The listing builds one solid part. Answer for the finished solid, in the listing's coordinates (mm). Round coordinates to 2 decimals unless told otherwise and drop trailing zeros. Loops run counter-clockwise (first coordinate to the right, second up) from the corner with the lowest first, then second, coordinate; pieces in that order, holes last. Notation, with made-up numbers: M 75,-14.5 L 93,-14.5 A12 ccw 93,-4.5 Z; hole C 47,88.25 d1. An arc over 180 degrees is marked long. Answer as a JSON object with one key per item and string values.
```python
from build123d import *

# Parameters (mm, degrees)
SKETCH1_W               = 10
SKETCH1_H               = 6
BOSS_EXTRUDE1_DEPTH     = 250
SKETCH3_R               = 3
CUT_EXTRUDE2_DEPTH      = 249
CUT_EXTRUDE2_DEPTH_BACK = 249
SKETCH2_W               = 8
SKETCH2_H               = 4
CUT_EXTRUDE4_DEPTH      = 251
CUT_EXTRUDE4_DEPTH_BACK = 1
SKETCH7_R               = 6
BOSS_EXTRUDE2_DEPTH     = 10
SKETCH9_R               = 5
CUT_EXTRUDE7_DEPTH      = 1
CUT_EXTRUDE7_DEPTH_BACK = 11


with BuildPart() as part:
    # Sketch1 → Boss-Extrude1 (new body)
    with BuildSketch(Plane.XY):
        Rectangle(SKETCH1_W, SKETCH1_H)
    extrude(amount=BOSS_EXTRUDE1_DEPTH)

    # Sketch3 → Cut-Extrude2 (cut, two sides)
    with BuildSketch(Plane(origin=(0, 0, 0), x_dir=(1, 0, 0), z_dir=(0, 1, 0))) as cut_extrude2_sk:
        with Locations((0, -245)):
            Circle(SKETCH3_R)
    extrude(amount=CUT_EXTRUDE2_DEPTH, mode=Mode.SUBTRACT)
    extrude(cut_extrude2_sk.sketch, amount=-CUT_EXTRUDE2_DEPTH_BACK, mode=Mode.SUBTRACT)

    # Sketch2 → Cut-Extrude4 (cut, two sides)
    with BuildSketch(Plane.XY) as cut_extrude4_sk:
        Rectangle(SKETCH2_W, SKETCH2_H)
    extrude(amount=CUT_EXTRUDE4_DEPTH, mode=Mode.SUBTRACT)
    extrude(cut_extrude4_sk.sketch, amount=-CUT_EXTRUDE4_DEPTH_BACK, mode=Mode.SUBTRACT)

    # Sketch7 → Boss-Extrude2 (add)
    with BuildSketch(Plane.ZY.offset(5)):
        with Locations((5, 0)):
            Circle(SKETCH7_R)
    extrude(amount=-BOSS_EXTRUDE2_DEPTH)

    # Sketch9 → Cut-Extrude7 (cut, two sides)
    with BuildSketch(Plane.ZY.offset(5)) as cut_extrude7_sk:
        with Locations((5, 0)):
            Circle(SKETCH9_R)
    extrude(amount=CUT_EXTRUDE7_DEPTH, mode=Mode.SUBTRACT)
    extrude(cut_extrude7_sk.sketch, amount=-CUT_EXTRUDE7_DEPTH_BACK, mode=Mode.SUBTRACT)


solid = part.part
```
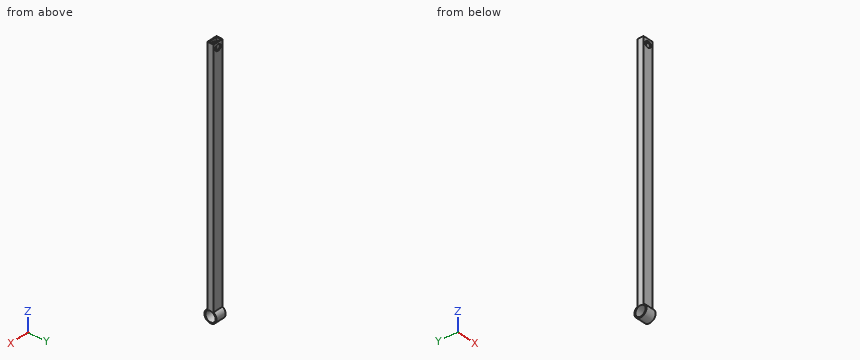
Item 1: The part is cut by section C-C (y = 0). Give the vertices of the cut face in (x, z), then the cut area to 3 significant figures.
Values follow:
{"outline": "M -5,-1 L 5,-1 L 5,0 L -5,0 Z; M -5,10 L 5,10 L 5,250 L 4,250 L 4,11 L -4,11 L -4,250 L -5,250 Z", "area": "498 mm^2"}
Item 2: The part is cut by section D-D (z = 245). Give the vertices of the cut face in (x, y), then the cut area to 3 significant figures.
Values follow:
{"outline": "M -5,-3 L -3,-3 L -3,-2 L -4,-2 L -4,2 L -3,2 L -3,3 L -5,3 Z; M 3,-3 L 5,-3 L 5,3 L 3,3 L 3,2 L 4,2 L 4,-2 L 3,-2 Z", "area": "16.0 mm^2"}
Item 3: The part is cut by section B-B (z = 184). Give the vertices of the cut face in (x, y).
Values follow:
{"outline": "M -5,-3 L 5,-3 L 5,3 L -5,3 Z; hole M -4,-2 L 4,-2 L 4,2 L -4,2 Z"}
Item 4: Straight lines are drawn through the part: line 1 (Y direction, x = 2.25, z = 86.5); line 2 (X direction, y = -2.65, z = 245); line 3 (X direction, y = 0, z = 154.5). For each, find the intervals that lie inside material, in ascending order.
Values follow:
{"line 1": "-3 to -2, 2 to 3", "line 2": "-5 to -3, 3 to 5", "line 3": "-5 to -4, 4 to 5"}
Item 5: The part is cut by section A-A (x = 0). Give the vertices of the cut face in (y, z).
Values follow:
{"outline": "M -3,10.2 A6 ccw long 3,10.2 L 3,242 L 2,242 L 2,10.66 A6 ccw -2,10.66 L -2,242 L -3,242 Z; M -3,248 L -2,248 L -2,250 L -3,250 Z; M 2,248 L 3,248 L 3,250 L 2,250 Z; hole C 0,5 d10"}
Item 6: Flat-ended cylindrical pins translate along their axes: P1, Ø1, axis at x = 4, y = -1, coming from the -Z side; P2, Ø5.5, axis at x = 0, z = 245, coming from the -Y side; P3, Ø4, axis at x = 1.5, z = 91, coming from the -Y side; P4, Ø1.5, axis at x = 0, z = 205.5, coming from the +Y side. Find the tip coordinate at first contact, or state that the pin passes through.
Values follow:
{"P1": "z = -0.98", "P2": "through", "P3": "y = -3", "P4": "y = 3"}
